Source: CAD feature listing. Evaluate the final solid. Frame: model axes, mm. A direction names the side the tool comes from. Give positions to 0.01 mm unless a question says otherwise; leave off trailing zeros. Write each loop counter-clockwise with the first axis right and the second up, starting at its lowest first coordinate (ties: lowest second). Pieces come first, ordered by that corner, then holes. Notation, with made-up numbers: (10.5, 43.5) -> (53.5, 43.5) arc R5 ccw to (53.5, 47.5) -> close; hole circle Ø9 at (67, -36.75). An arc over 180 degrees is marked (long way). Use a Markdown table: item, result. Add a question column.
```python
from build123d import *

# Parameters (mm, degrees)
BOSS_EXTRU_1_DEPTH      = 30
ESQUISSE2_W             = 110
ESQUISSE2_H             = 15
ENL_V_MAT_EXTRU_1_DEPTH = 30
ENL_V_START             = -10
ESQUISSE3_W             = 44.19
ESQUISSE3_H             = 7.5
ENL_V_MAT_EXTRU_2_DEPTH = 10
ESQUISSE4_W             = 5
ESQUISSE4_H             = 7.5
BOSS_EXTRU_2_DEPTH      = 10
ESQUISSE5_W             = 7.5
ESQUISSE5_H             = 3
BOSS_EXTRU_3_DEPTH      = 6
ESQUISSE6_W             = 7.5
ESQUISSE6_H             = 3
BOSS_EXTRU_4_DEPTH      = 5.5
CONG_1_R                = 10


with BuildPart() as part:
    # Esquisse1 → Boss.-Extru.1 (new body)
    with BuildSketch(Plane.XY):
        with BuildLine():
            Line((-55, 10), (55, 10))
            ThreePointArc((55, 10), (65, 0), (55, -10))
            Line((55, -10), (-55, -10))
            ThreePointArc((-55, -10), (-65, 0), (-55, 10))
        make_face()
        with BuildLine():
            Line((-55, 1.5), (55, 1.5))
            ThreePointArc((55, 1.5), (56.5, 0), (55, -1.5))
            Line((55, -1.5), (-55, -1.5))
            ThreePointArc((-55, -1.5), (-56.5, 0), (-55, 1.5))
        make_face(mode=Mode.SUBTRACT)
    extrude(amount=BOSS_EXTRU_1_DEPTH)

    # Esquisse2 → Enlèv. mat.-Extru.1 (cut)
    with BuildSketch(Plane(origin=(0, 10, 0), x_dir=(1, 0, 0), z_dir=(0, 1, 0))):
        with Locations((0, -15)):
            Rectangle(ESQUISSE2_W, ESQUISSE2_H)
    extrude(amount=-ENL_V_MAT_EXTRU_1_DEPTH, mode=Mode.SUBTRACT)

    # Esquisse3 → Enlèv. mat.-Extru.2 (cut)
    with BuildSketch(Plane(origin=(0, 10, 0), x_dir=(1, 0, 0), z_dir=(0, 1, 0)).offset(ENL_V_START)):
        with Locations((0, -26.25)):
            Rectangle(ESQUISSE3_W, ESQUISSE3_H)
    extrude(amount=-ENL_V_MAT_EXTRU_2_DEPTH, mode=Mode.SUBTRACT)

    # Esquisse4 → Boss.-Extru.2 (add)
    with BuildSketch(Plane(origin=(0, -1.5, 0), x_dir=(1, 0, 0), z_dir=(0, 1, 0))):
        with Locations((-24.595, -26.25)):
            Rectangle(ESQUISSE4_W, ESQUISSE4_H)
        with Locations((24.595, -26.25)):
            Rectangle(ESQUISSE4_W, ESQUISSE4_H)
    extrude(amount=BOSS_EXTRU_2_DEPTH)

    # Esquisse5 → Boss.-Extru.3 (add)
    with BuildSketch(Plane(origin=(27.095, 0, 0), x_dir=(0, 0, -1), z_dir=(1, 0, 0))):
        with Locations((-26.25, 0)):
            Rectangle(ESQUISSE5_W, ESQUISSE5_H)
    extrude(amount=BOSS_EXTRU_3_DEPTH)

    # Esquisse6 → Boss.-Extru.4 (add)
    with BuildSketch(Plane.ZY.offset(27.095)):
        with Locations((26.25, 0)):
            Rectangle(ESQUISSE6_W, ESQUISSE6_H)
    extrude(amount=BOSS_EXTRU_4_DEPTH)

    # Congé1
    cong_1_edges = [part.edges().sort_by_distance(p)[0] for p in [
        (22.095, -10, 26.25),
        (-22.095, -10, 26.25),
    ]]
    fillet(cong_1_edges, radius=CONG_1_R)


solid = part.part
```
(1) Mould query, pull axis Z, two halves, no side actions, for faces 6 (the flat face through (1, -2, 0)), 7 (the flat face through (-43, -10, 26)), 8 (the flat face through (-1, -6, 7.5)). Classes: +Z half, -Z half, draft (parallel to the pull), parting line (faces both ways), or undercut.
(2) Cut plane D-D on x = -31. Return the cut outline in (y, z).
(3) Cut plane C-C on y = -5.75. Return the cut outline in (x, z).
(4) Material intervals for L1, parallel to Z at x = 30.5, y = -3.5; L2, parallel to Y at x = -15.5, z = 5.75; L3, parallel to Z at x = 21, y = -1.75, sorted ascending.
(5) First-contact query: pin 1 Ø7 at (y, z) = (8, 11.5) entering from -X; pin 2 Ø1.2 at (y, z) = (0.5, 27) entering from -X; pin 3 Ø6 at (y, z) = (-6.5, 13) entering from +X; pin 4 Ø6 at (y, z) = (8, 5.5) entering from -X. Flat tips, straight axial feed; report the tip coordinate or a pass-through.
(6) Cut plane B-B on x = -49. Return the cut outline in (y, z).
(7) Access query for faces 1 (the flat face through (1, -1.5, 4)), 2 (the flat face through (55, -6, 15)), 3 (the cylindrical face through (-25.102, -7.148, 26.197)), 4 (the flat face through (44, -10, 26)), 5 (the cylindrical face through (56.5, 0, 14.8)). Directions: +Z, -Z, +X, -X, +Y, -Y. A direction counts if a zero-diameter tool reaches every point of the face in a straight line with its end or side. Return the directions, or none.
(8) Cut plane A-A on z = 20.5. Return the cut outline in (x, y).
Output:
| question | item | result |
|---|---|---|
| 1 | face 6 | -Z half |
| 1 | face 7 | draft |
| 1 | face 8 | undercut |
| 2 | outline | (-10, 0) -> (-1.5, 0) -> (-1.5, 7.5) -> (-10, 7.5) -> close; (-9.94, 22.5) -> (10, 22.5) -> (10, 30) -> (-9.94, 30) -> close; (1.5, 0) -> (10, 0) -> (10, 7.5) -> (1.5, 7.5) -> close |
| 3 | outline | (-63.18, 0) -> (63.18, 0) -> (63.18, 30) -> (23.91, 30) -> (23.91, 22.5) -> (55, 22.5) -> (55, 7.5) -> (-55, 7.5) -> (-55, 22.5) -> (-23.91, 22.5) -> (-23.91, 30) -> (-63.18, 30) -> close |
| 4 | L1 | 0 to 7.5, 22.5 to 30 |
| 4 | L2 | -10 to -1.5, 1.5 to 10 |
| 4 | L3 | 0 to 7.5 |
| 5 | pin 1 | x = -63.93 |
| 5 | pin 2 | x = -65 |
| 5 | pin 3 | x = 64.37 |
| 5 | pin 4 | x = -63.66 |
| 6 | outline | (-10, 0) -> (-1.5, 0) -> (-1.5, 7.5) -> (-10, 7.5) -> close; (-10, 22.5) -> (-1.5, 22.5) -> (-1.5, 30) -> (-10, 30) -> close; (1.5, 0) -> (10, 0) -> (10, 7.5) -> (1.5, 7.5) -> close; (1.5, 22.5) -> (10, 22.5) -> (10, 30) -> (1.5, 30) -> close |
| 7 | face 1 | -Z |
| 7 | face 2 | +Y, -Y |
| 7 | face 3 | +Z, -Y |
| 7 | face 4 | +Z, -Z, +X, -X, -Y |
| 7 | face 5 | +Z, -Z |
| 8 | outline | (-55, -10) -> (-55, -1.5) arc R1.5 cw to (-55, 1.5) -> (-55, 10) arc R10 ccw to start; (55, -10) arc R10 ccw to (55, 10) -> (55, 1.5) arc R1.5 cw to (55, -1.5) -> close |
